Work out the finished part from the listing and answer in its coordinate system (mm). Face numbers are marked on the shaded views. Round coordinates to 2 decimals unless told otherwise and drop trailing zeros. Write each loop counter-clockwise with the first axis right and the second up, starting at its lowest first coordinate (ties: lowest second). Pieces come first, ordered by that corner, then holes. Notation, with made-up numbers: (35.25, 84.5) - (64.25, 84.5) arc R8 ccw to (64.25, 90.5) - close; hole circle Ø4 at (85, 34.5). An arc over 180 degrees is marked (long way). Answer as a JSON object with one key per item and string values.
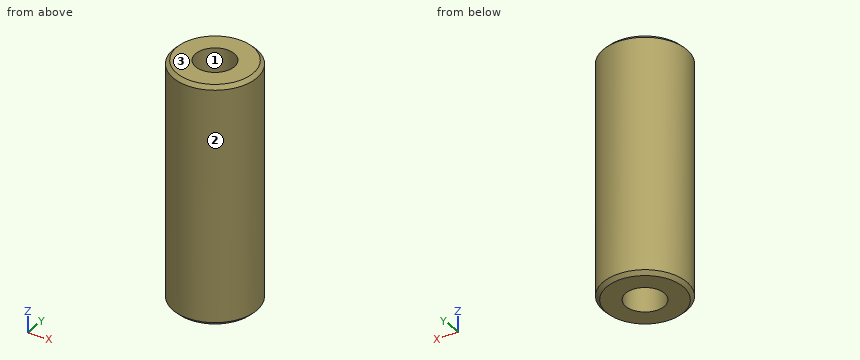
Autodesk Inventor part; units mm, degrees
ref_plane "YZ Plane" through (0, 0, 0) normal (1, 0, 0) x (0, 1, 0)
ref_plane "XZ Plane" through (0, 0, 0) normal (0, 1, 0) x (-1, 0, 0)
ref_plane "XY Plane" through (0, 0, 0) normal (0, 0, 1) x (1, 0, 0)
sketch "Skizze1" plane through (0, 0, 0) normal (0, 0, 1) x (1, 0, 0)
  circle A0 centre (0, 0) radius 3.5
  dimension "d0" = 7
extrude "Extrusion1" add sketch "Skizze1" along normal mid plane 20
chamfer "Fase1" distance 0.3 angle 45 2 edges at (-3.5, 0, 10) (-3.5, 0, -10)
hole "Bohrung1" at (0, 0, 10) direction (0, 0, -1) diameter 3.242 end through all
equation "\"d0\" = Durchmesser"
equation "\"d1\" = Länge"
equation "\"d9\" = Länge"
equation "\"Länge\" = 20"
equation "\"Durchmesser\" = 7"
properties part number "Distanzhülse_M4x20"
Item 1: A cutting plane is placed at C-C (z = -2.75). Write down the section's boundary in (x, y).
Results found:
{"outline": "circle Ø7 at (0, 0); hole circle Ø3.24 at (0, 0)"}
Item 2: Each of these flat-tipped pins is pushed along its axis until it touches: P1, Ø1.5, axis at y = -2.5, z = 1, coming from the +X side; P2, Ø1, axis at x = 2.5, z = 0, coming from the -Y side. Where does it stop, or does it pass through?
Results found:
{"P1": "x = 3.03", "P2": "y = -2.87"}
Item 3: Determine the mould class of the marked faces 1, 2 and 3 for opening direction X: pulls with the +X half, pulls with the -X half, needs draft (parallel to the pull), parting line crosses it, or undercut.
Results found:
{"face 1": "undercut", "face 2": "parting line crosses it", "face 3": "needs draft"}
Item 4: A cutting plane is placed at A-A (y = 0). Write down the section's boundary in (x, z), and give its area (3 significant figures).
Results found:
{"outline": "(-3.5, -9.7) - (-3.2, -10) - (-1.62, -10) - (-1.62, 10) - (-3.2, 10) - (-3.5, 9.7) - close; (1.62, -10) - (3.2, -10) - (3.5, -9.7) - (3.5, 9.7) - (3.2, 10) - (1.62, 10) - close", "area": "75.0 mm²"}
Item 5: Consider line 1 along Y through (x, z) = (0, -5); line 2 along X through (y, z) = (0.5, -0.75); line 3 along X through (y, z) = (0.25, -1.5). Determine where each line is inside the solid, lowest interval first.
Results found:
{"line 1": "-3.5 to -1.62, 1.62 to 3.5", "line 2": "-3.46 to -1.54, 1.54 to 3.46", "line 3": "-3.49 to -1.6, 1.6 to 3.49"}
